Could you check a few things on this drawing? It's one solid part, dimensions in mm from its lowest x, y, z. A direction names the side the tool comes from. Round coordinates to 2 decimals unless told otherwise and drop trailing zeros. Write each loop counter-clockwise with the first axis right and the second up, starting at its lowest first coordinate (ties: lowest second). Pieces come first, ordered by that corner, then holes. Notation, with made-up numbers: (55.25, -27.5) -> (112.25, -27.5) arc R13 cw to (112.25, -8.5) -> close; hole circle Ø4 at (30.25, 36.25). An arc over 180 degrees is marked (long way). Put each result on its own line as item: value. Start each with the question number.
1) I want a section at D-D, the plane x = 19. List the corners of the cut face in (y, z) for me.
2) Which directions (+Z, -Z, +X, -X, +Y, -Y) give clear straight access to the entire face, cutting with the end or side of a thin tool? Please do the marked faces 1 and 2.
3) If I drill on line 1 along Y through (x, z) = (4.5, 23.25); line 2 along X through (y, z) = (39, 13.5) (1 decimal); line 3 along Y through (x, z) = (14.5, 20.5), over which ranges is the centre line in solid material (lowest first)? Write a range as [from, to].
4) I want a section at C-C, the plane y = 55. List the corners of the cut face in (x, z) for me (1 decimal).
5) We'd pull the mould along X, two halves only. Please class the marked faces 3, 4 and 5: released by +X, released by -X, zero draft, split by the parting line, or undercut.
6) I want a section at B-B, the plane y = 77.5. Give the number of separate pieces and of enclosed holes in the cut face, then the cut area to 3 significant figures.
7) I want a section at A-A, the plane x = 35.5. List the corners of the cut face in (y, z) for me.
8) Will these pins go through, and if not, where does the flat tip stop? P1, Ø10, axis at x = 20, z = 19.5, coming from the +Y side; P2, Ø12, axis at x = 27, z = 13.5, coming from the -Y side; P3, Ø5, axis at y = 73, z = 11, coming from the +X side.
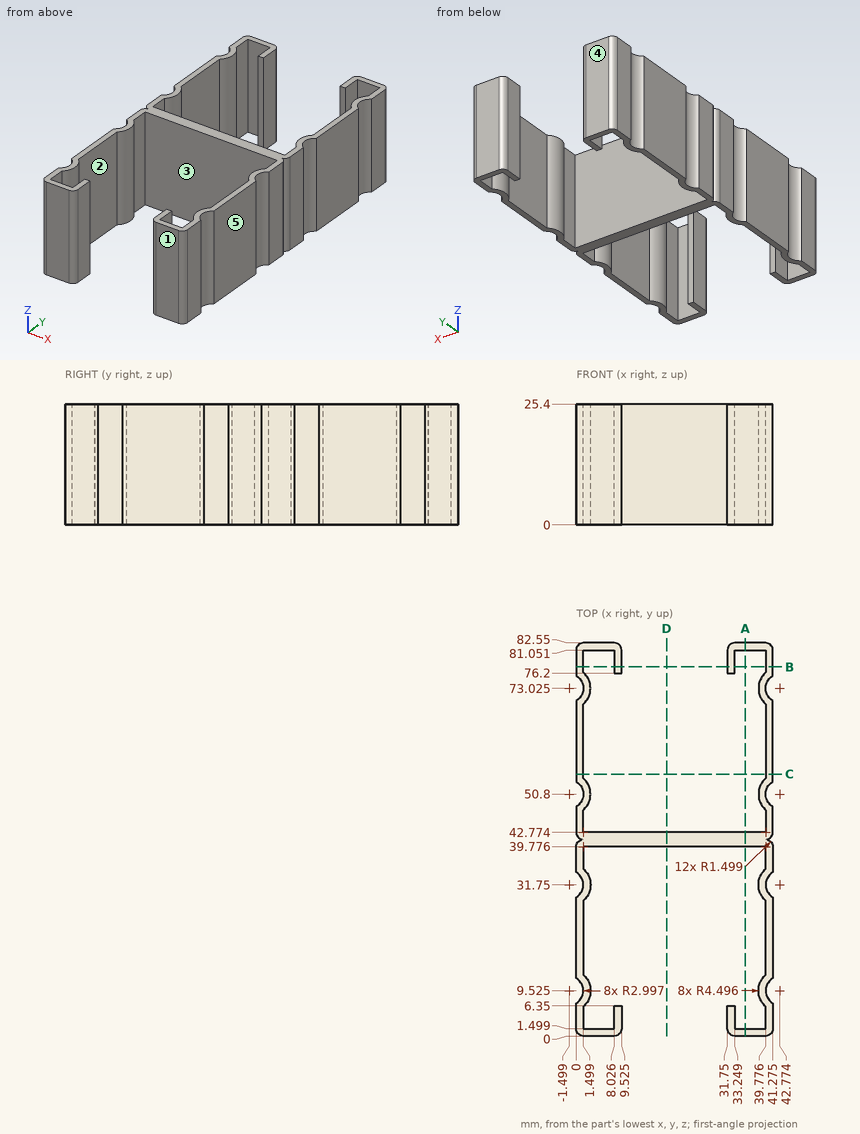
Findings:
1. outline: (39.78, 0) -> (42.77, 0) -> (42.77, 25.4) -> (39.78, 25.4) -> close
2. face 1: +Z, -Z, +X, -X, -Y
2. face 2: +Z, -Z
3. line 1: y = [0, 1.5], [39.78, 42.77], [81.05, 82.55]
3. line 2: x = [0, 1.5], [39.8, 41.3]
3. line 3: y = [39.78, 42.77]
4. outline: (0, 0) -> (1.5, 0) -> (1.5, 25.4) -> (0, 25.4) -> close; (39.8, 0) -> (41.3, 0) -> (41.3, 25.4) -> (39.8, 25.4) -> close
5. face 3: undercut
5. face 4: zero draft
5. face 5: released by +X
6. separate pieces: 4
6. enclosed holes: 0
6. area: 152 mm2
7. outline: (0, 0) -> (1.5, 0) -> (1.5, 25.4) -> (0, 25.4) -> close; (39.78, 0) -> (42.77, 0) -> (42.77, 25.4) -> (39.78, 25.4) -> close; (81.05, 0) -> (82.55, 0) -> (82.55, 25.4) -> (81.05, 25.4) -> close
8. P1: stops at y = 42.77
8. P2: stops at y = 0.02
8. P3: stops at x = 41.16
